The drawing under review shows one solid part. Ordinate dimensions are in mm from its lowest x, y, z. Round coordinates to 2 decimals unless told otherwise and drop trailing zeros. Loops run counter-clockwise (first coordinate to the right, second up) from the corner with the lowest first, then second, coordinate; pieces in that order, holes last. Notation, with made-up numbers: M -27.75,26.5 L -9.75,26.5 A20 cw -9.75,63.5 Z; hole C 9,21 d5. An arc over 180 degrees is marked long. Use a Markdown table: item, result.
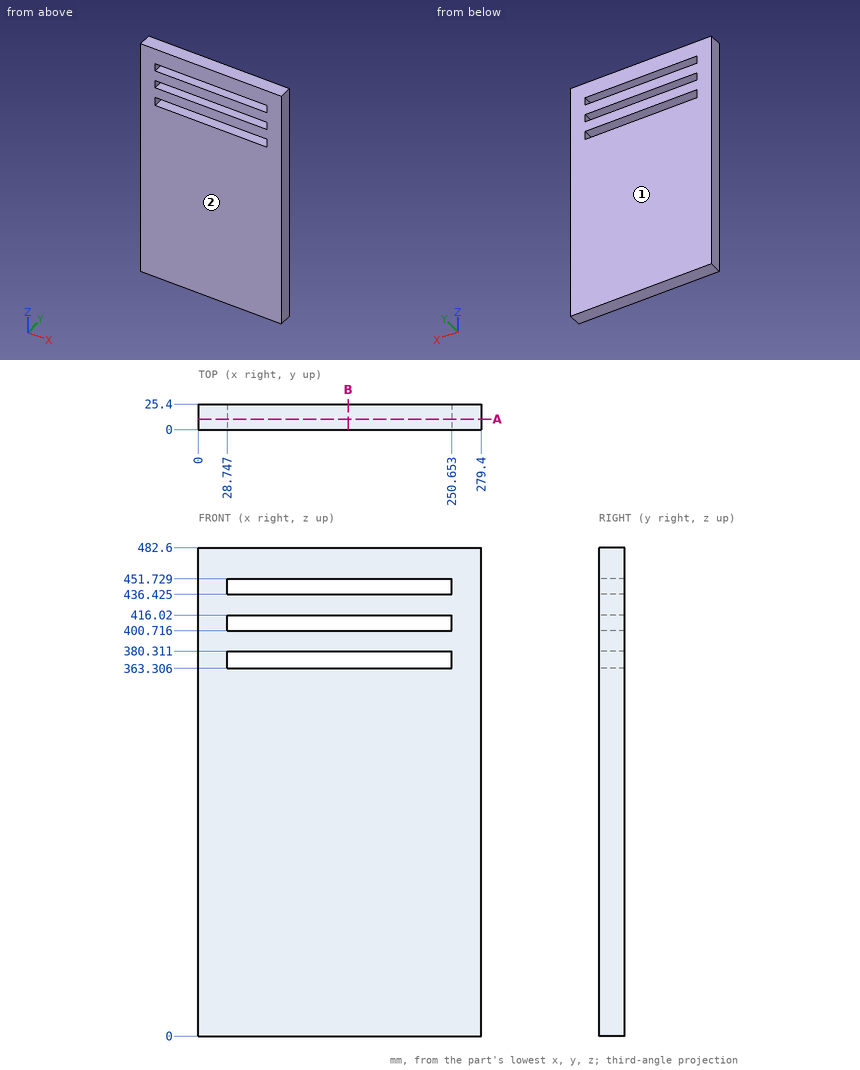
1. Take a section at A-A on y = 10.5. Give the boundary of the cut face in (x, z) (1 decimal).
Check values:
| item | result |
|---|---|
| outline | M 0,0 L 279.4,0 L 279.4,482.6 L 0,482.6 Z; hole M 28.7,363.3 L 250.7,363.3 L 250.7,380.3 L 28.7,380.3 Z; hole M 28.7,400.7 L 250.7,400.7 L 250.7,416 L 28.7,416 Z; hole M 28.7,436.4 L 250.7,436.4 L 250.7,451.7 L 28.7,451.7 Z |
2. Take a section at B-B on x = 148. Give the boundary of the cut face in (y, z) (1 decimal), and give its area (3 significant figures).
Check values:
| item | result |
|---|---|
| outline | M 0,0 L 25.4,0 L 25.4,363.3 L 0,363.3 Z; M 0,380.3 L 25.4,380.3 L 25.4,400.7 L 0,400.7 Z; M 0,416 L 25.4,416 L 25.4,436.4 L 0,436.4 Z; M 0,451.7 L 25.4,451.7 L 25.4,482.6 L 0,482.6 Z |
| area | 11,000 mm² |
3. The part is to be moulded in two halves that separate along Y. For the marked faces 1 and 2, say which applies: pulls with the +Y half, pulls with the -Y half, needs draft (parallel to the pull), parting line crosses it, or undercut.
Check values:
| item | result |
|---|---|
| face 1 | pulls with the +Y half |
| face 2 | pulls with the -Y half |
4. Wall thickness on line 1 along Z through (x, y) = (231.5, 16.25) (1 decimal); line 2 along X through (y, z) = (12, 364): over which ranges is each line inside the solid? List them lowest first. Write a range as from..to.
Check values:
| item | result |
|---|---|
| line 1 | z = 0..363.3, 380.3..400.7, 416..436.4, 451.7..482.6 |
| line 2 | x = 0..28.75, 250.65..279.4 |
